from build123d import *

# Parameters (mm, degrees)
SKETCH1_W           = 53.52
SKETCH1_H           = 25.42
BOSS_EXTRUDE2_DEPTH = 12.06
SKETCH2_R           = 5.05
BOSS_EXTRUDE3_DEPTH = 8.33
SKETCH3_R           = 4.745
BOSS_EXTRUDE4_DEPTH = 12
SKETCH4_R           = 4.745
BOSS_EXTRUDE5_DEPTH = 87.4
FILLET1_R           = 4.318
FILLET2_R           = 1.27
FILLET3_R           = 1.27


with BuildPart() as part:
    # Sketch1 → Boss-Extrude2 (new body)
    with BuildSketch(Plane(origin=(0, 0, 0), x_dir=(1, 0, 0), z_dir=(0, 1, 0))):
        with Locations((0.655882353, 2.019117647)):
            Rectangle(SKETCH1_W, SKETCH1_H)
    extrude(amount=BOSS_EXTRUDE2_DEPTH)

    # Sketch2 → Boss-Extrude3 (add)
    with BuildSketch(Plane(origin=(27.415882353, 0, 0), x_dir=(0, 0, -1), z_dir=(1, 0, 0))):
        with Locations(Location((8.151317647, 7.5138, 0), (0, 0, 115.810680581))):
            Circle(SKETCH2_R)
    extrude(amount=BOSS_EXTRUDE3_DEPTH)

    # Sketch3 → Boss-Extrude4 (add)
    with BuildSketch(Plane(origin=(35.745882353, 0, 0), x_dir=(0, 0, -1), z_dir=(1, 0, 0))):
        with Locations((8.151317647, 7.5138)):
            Circle(SKETCH3_R)
    extrude(amount=BOSS_EXTRUDE4_DEPTH)

    # Sketch4 → Boss-Extrude5 (add)
    with BuildSketch(Plane(origin=(47.745882353, 0, 0), x_dir=(0, 0, -1), z_dir=(1, 0, 0))):
        with Locations((8.151317647, 7.5138)):
            Circle(SKETCH4_R)
    extrude(amount=BOSS_EXTRUDE5_DEPTH)

    # Fillet1
    fillet1_edges = [part.edges().sort_by_distance(p)[0] for p in [
        (135.145882353, 7.5138, -3.406317647),
    ]]
    fillet(fillet1_edges, radius=FILLET1_R)

    # Fillet2
    fillet2_edges = [part.edges().sort_by_distance(p)[0] for p in [
        (0.655882353, 0, 10.690882353),
        (0.655882353, 12.06, 10.690882353),
        (27.415882353, 6.03, 10.690882353),
        (-26.104117647, 6.03, 10.690882353),
    ]]
    fillet(fillet2_edges, radius=FILLET2_R)

    # Fillet3
    fillet3_edges = [part.edges().sort_by_distance(p)[0] for p in [
        (0.655882353, 12.06, -14.729117647),
        (0.655882353, 0, -14.729117647),
        (-26.104117647, 6.03, -14.729117647),
        (27.415882353, 6.03, -14.729117647),
    ]]
    fillet(fillet3_edges, radius=FILLET3_R)


solid = part.part
Here's how the part is built. I have some questions about the finished solid (model axes, mm). A direction names the side the tool comes from. Give positions to 0.01 mm unless a question says otherwise; leave off trailing zeros. Order: outer loops, then holes, each group sorted by start corner. A loop starts at its lowest first (then second) coordinate and runs counter-clockwise, first axis right, second up. Notation, with made-up numbers: (6.5, 22) -> (64.5, 22) arc R27 cw to (64.5, 50) -> close; hole circle Ø7 at (-37.75, 29). An arc over 180 degrees is marked (long way). One line per item, written item: value. Start each with the question number.
1. I need wall thicknesses on probe 1 along Y at (x, z) = (-12, -12.75); probe 2 along X at (y, z) = (1.75, -13.5); probe 3 along Z at (x, y) = (103.5, 7.25). Which ranges of each line are inside material? Lowest first, please. Write a range as from..to.
2. Imagine slicing it at C-C, the plane x = 116. List the corners of the cut face in (y, z) for me (3 decimals), plus the area to 3 significant figures.
3. For faces 1 (the face through (82.621, 8.939, -12.677)), 2 (the face through (0, 0, -2)), 3 (the face through (0, 12.06, -2)), which set-ups out of +Z, -Z, +X, -X, +Y, -Y let a thin tool reach every point of the face, with its end or its side?
4. Imagine slicing it at A-A, the plane x = 7. List the corners of the cut face in (y, z) for me, plus the area to 3 significant figures.
5. Will these pins go through, and if not, where does the flat tip stop? pin 1 Ø1.5 at (y, z) = (8, 2) entering from +X; pin 2 Ø1 at (x, y) = (58.5, 7) entering from +Z; pin 3 Ø0.6 at (y, z) = (12.5, -8.5) entering from -X.
6. Imagine slicing it at B-B, the plane z = 1. List the corners of the cut face in (x, y) for me.
Values follow:
1. probe 1: y = 0..12.06
1. probe 2: x = -26.1..27.42
1. probe 3: z = -12.89..-3.41
2. outline: circle Ø9.49 at (7.514, -8.151)
2. area: 70.7 mm2
3. face 1: +X
3. face 2: +Z, -Z, +X, -X, -Y
3. face 3: +Z, -Z, -X, +Y
4. outline: (0, -13.46) arc R1.27 ccw to (1.27, -14.73) -> (10.79, -14.73) arc R1.27 ccw to (12.06, -13.46) -> (12.06, 9.42) arc R1.27 ccw to (10.79, 10.69) -> (1.27, 10.69) arc R1.27 ccw to (0, 9.42) -> close
4. area: 305 mm2
5. pin 1: stops at x = 27.42
5. pin 2: stops at z = -3.41
5. pin 3: stops at x = 27.42
6. outline: (-26.1, 0) -> (27.42, 0) -> (27.42, 12.06) -> (-26.1, 12.06) -> close
